Answer from the drawing. Dimensions are ordinates in mm from the lowest x, y and z of the part. Give positions to 0.01 mm unless a question says otherwise; leave off trailing zeros. Order: outer loops, then holes, each group sorted by start corner. A loop starts at its lowest first (then second) coordinate and runs counter-clockwise, first axis right, second up.
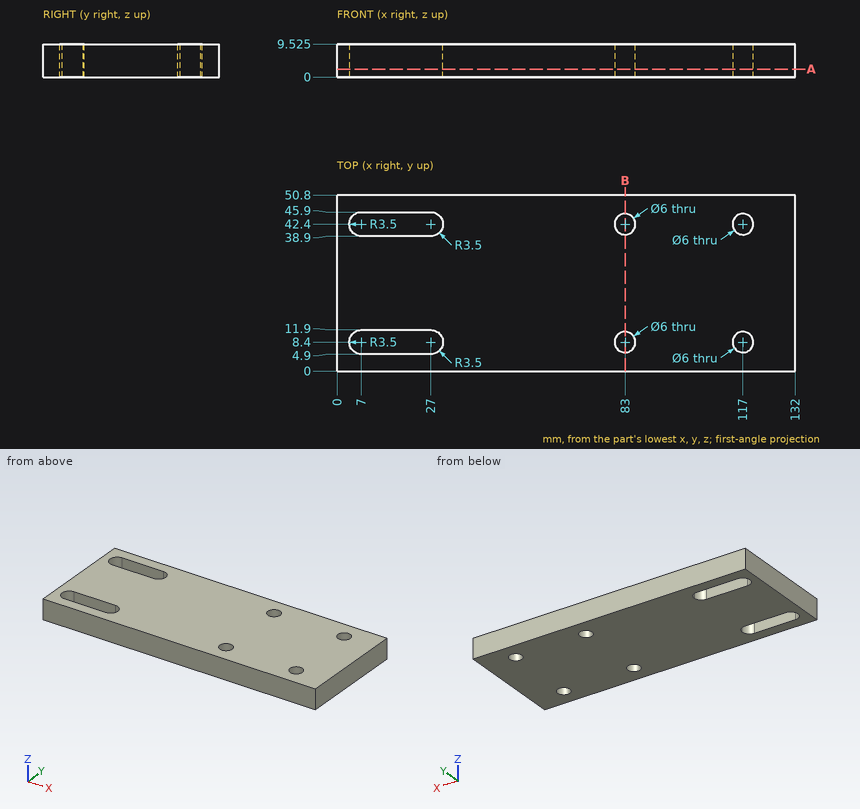
1) Given pin 1 (1.5 mm diameter, centred on x = 66.5, y = 27, fed in from -Z); pin 2 (3.5 mm diameter, centred on x = 117, y = 8.4, fed in from +Z), each flat-ended and moving along its own axis, determine where each tip first touches the part or whether it passes through.
Final values:
pin 1: stops at z = 0
pin 2: passes through
2) The part is cut by section B-B on x = 83. Determine the outline of the cut face in (y, z) (3 decimals), and give its area (3 significant figures).
Final values:
outline: (0, 0) - (5.4, 0) - (5.4, 9.525) - (0, 9.525) - close; (11.4, 0) - (39.4, 0) - (39.4, 9.525) - (11.4, 9.525) - close; (45.4, 0) - (50.8, 0) - (50.8, 9.525) - (45.4, 9.525) - close
area: 370 mm2
3) The part is cut by section A-A on z = 2.25. Determine the outline of the cut face in (x, y), and give its area (3 significant figures).
Final values:
outline: (0, 0) - (132, 0) - (132, 50.8) - (0, 50.8) - close; hole (7, 4.9) - (27, 4.9) arc R3.5 ccw to (30.5, 8.4) arc R3.5 ccw to (27, 11.9) - (7, 11.9) arc R3.5 ccw to start; hole (7, 38.9) - (27, 38.9) arc R3.5 ccw to (30.5, 42.4) arc R3.5 ccw to (27, 45.9) - (7, 45.9) arc R3.5 ccw to start; hole circle Ø6 at (83, 8.4); hole circle Ø6 at (83, 42.4); hole circle Ø6 at (117, 8.4); hole circle Ø6 at (117, 42.4)
area: 6,240 mm2
4) Consider L1, parallel to Y at x = 83, z = 3.75; L2, parallel to Y at x = 8, z = 5.5. Determine where each line is inside the solid, lowest interval first.
Final values:
L1: y = 0 to 5.4, 11.4 to 39.4, 45.4 to 50.8
L2: y = 0 to 4.9, 11.9 to 38.9, 45.9 to 50.8
